Read the model definition and answer for the solid it produces. Units are mm, in the model's axes. A direction names the side the tool comes from. Coordinates: 2 decimals unless noted, no trailing zeros. Write each loop counter-clockwise with the first axis right and the second up, starting at its lowest first coordinate (ties: lowest second). Pieces come first, ordered by that corner, then holes.
1) The part is cut by section A-A (x = 234). Determine the outline of the cut face in (y, z).
2) Which of the six approach directions +Z, -Z, +X, -X, +Y, -Y give full straight-line access (tool end or side, diameter ignored) to faces 1 (the face through (70, 3, -242)), 2 (the face through (138, 3, -257))?
3) Each of these flat-tipped pins is pushed along its axis until it touches: pin 1 Ø1.6 at (x, z) = (4, -129.5) entering from +Y; pin 2 Ø1.7 at (x, z) = (140, -4) entering from -Y. Where does it stop, or does it pass through?
4) Find the intervals of material crossed by line 1 (X direction, y = 5.15, z = -128.5); line 2 (Z direction, x = 205, y = 5.6); line 3 (Z direction, x = 140, y = 1.75), in increasing order.
5) Determine the mould class of faces 3 (the face through (138, 0, -130)), 4 (the face through (70, 3, -15)), 5 (the face through (280, 3, -127)) for opening direction X: +X half, -X half, draft (parallel to the pull), parting line (faces both ways), or undercut.
from build123d import *

# Parameters (mm, degrees)
SKETCH1_W           = 280
SKETCH1_H           = 257
BOSS_EXTRUDE2_DEPTH = 6
SKETCH3_R           = 1.45
CUT_EXTRUDE1_DEPTH  = 381.111825651
SKETCH4_R           = 2.7
CUT_EXTRUDE4_DEPTH  = 2.5
SKETCH8_W           = 60
SKETCH8_H           = 10
CUT_EXTRUDE5_DEPTH  = 3


with BuildPart() as part:
    # Sketch1 → Boss-Extrude2 (new body)
    with BuildSketch(Plane(origin=(0, 0, 0), x_dir=(1, 0, 0), z_dir=(0, 1, 0))):
        with Locations((140, 128.5)):
            Rectangle(SKETCH1_W, SKETCH1_H)
    extrude(amount=BOSS_EXTRUDE2_DEPTH)

    # Sketch3 → Cut-Extrude1 (cut, through all)
    with BuildSketch(Plane(origin=(0, 6, 0), x_dir=(1, 0, 0), z_dir=(0, 1, 0))):
        with Locations(Location((4.002224382, 252.997775618, 0), (0, 0, 270))):
            Circle(SKETCH3_R)
        with Locations(Location((275.997775618, 252.997775618, 0), (0, 0, 270))):
            Circle(SKETCH3_R)
        with Locations(Location((4.002224382, 4.002224382, 0), (0, 0, 270))):
            Circle(SKETCH3_R)
        with Locations(Location((275.997775618, 4.002224382, 0), (0, 0, 270))):
            Circle(SKETCH3_R)
        with Locations(Location((4.002224382, 128.5, 0), (0, 0, 270))):
            Circle(SKETCH3_R)
        with Locations(Location((275.997775618, 128.5, 0), (0, 0, 270))):
            Circle(SKETCH3_R)
        with Locations(Location((140, 4.002224382, 0), (0, 0, 270))):
            Circle(SKETCH3_R)
        with Locations(Location((140, 252.997775618, 0), (0, 0, 270))):
            Circle(SKETCH3_R)
    extrude(amount=-CUT_EXTRUDE1_DEPTH, mode=Mode.SUBTRACT)

    # Sketch4 → Cut-Extrude4 (cut)
    with BuildSketch(Plane(origin=(0, 6, 0), x_dir=(1, 0, 0), z_dir=(0, 1, 0))):
        with Locations(Location((4.002224382, 4.002224382, 0), (0, 0, 270))):
            Circle(SKETCH4_R)
        with Locations(Location((4.002224382, 252.997775618, 0), (0, 0, 270))):
            Circle(SKETCH4_R)
        with Locations(Location((275.997775618, 252.997775618, 0), (0, 0, 270))):
            Circle(SKETCH4_R)
        with Locations(Location((275.997775618, 4.002224382, 0), (0, 0, 270))):
            Circle(SKETCH4_R)
        with Locations(Location((4.002224382, 128.5, 0), (0, 0, 270))):
            Circle(SKETCH4_R)
        with Locations(Location((275.997775618, 128.5, 0), (0, 0, 270))):
            Circle(SKETCH4_R)
        with Locations(Location((140, 252.997775618, 0), (0, 0, 270))):
            Circle(SKETCH4_R)
        with Locations(Location((140, 4.002224382, 0), (0, 0, 270))):
            Circle(SKETCH4_R)
    extrude(amount=-CUT_EXTRUDE4_DEPTH, mode=Mode.SUBTRACT)

    # Sketch8 → Cut-Extrude5 (cut)
    with BuildSketch(Plane(origin=(0, 6, 0), x_dir=(1, 0, 0), z_dir=(0, 1, 0))):
        with Locations((70, 242)):
            Rectangle(SKETCH8_W, SKETCH8_H)
        with Locations((70, 14.997514144)):
            Rectangle(SKETCH8_W, SKETCH8_H)
        with Locations((210, 14.997514144)):
            Rectangle(SKETCH8_W, SKETCH8_H)
        with Locations((210, 242)):
            Rectangle(SKETCH8_W, SKETCH8_H)
    extrude(amount=-CUT_EXTRUDE5_DEPTH, mode=Mode.SUBTRACT)


solid = part.part
Reported:
1. outline: (0, -257) - (6, -257) - (6, -247) - (3, -247) - (3, -237) - (6, -237) - (6, -20) - (3, -20) - (3, -10) - (6, -10) - (6, 0) - (0, 0) - close
2. face 1: +Y
2. face 2: -Z, +X, -X, +Y, -Y
3. pin 1: stops at y = 3.5
3. pin 2: passes through
4. line 1: x = 0 to 1.3, 6.7 to 273.3, 278.7 to 280
4. line 2: z = -257 to -247, -237 to -20, -10 to 0
4. line 3: z = -257 to -254.45, -251.55 to -5.45, -2.55 to 0
5. face 3: draft
5. face 4: undercut
5. face 5: +X half
